Verification items for the finished model (mm, model axes). A direction names the side the tool comes from. Coordinates: 2 decimals unless noted, no trailing zeros. Order: outer loops, then holes, each group sorted by start corner. A loop starts at its lowest first (then second) coordinate and runs counter-clockwise, first axis right, second up. Notation, with made-up numbers: M 34.5,-11.5 L 61.5,-11.5 A8 ccw 61.5,-2.5 Z; hole C -30,74.5 d5. An arc over 180 degrees is marked long. Return JSON: item names as keys, results as strings. Group by question number.
1. Material ranges on line 1 along Y through (x, z) = (0, 12.15); line 2 along X through (y, z) = (4, 2.25); line 3 along X through (y, z) = (0, 11.5), recorded low to high.
2. Section check D-D, the plane z = 10. Record the cut outline in (x, y), plus the area to 3 significant figures.
3. Gauge pin test, flat ends, axial feed: pin 1 (2.5 mm diameter, centred on y = 0, z = 7.5, fed in from -X); pin 2 (2 mm diameter, centred on x = -3.5, z = 11.5, fed in from +Y); pin 3 (1.5 mm diameter, centred on x = -2, y = 8, fed in from +Z). Record the tip position at first contact, or that the pin passes through.
4. Section check A-A, the plane y = 0. Record the cut outline in (x, z), plus the area to 3 significant figures.
5. Section check C-C, the plane z = 7. Record the cut outline in (x, y).
6. Mould release check, pull along X, two halves, no side actions. Record for faces 1 (the conical face through (1.409, 3.399, 12.636)), 2 (the flat face through (1.3, 1.3, 13)), 3 (the flat face through (1.361, -2.314, 7.479)): +X half, -X half, draft (parallel to the pull), parting line (faces both ways), or undercut.
7. Section check B-B, the plane z = 1.75. Record the cut outline in (x, y).
8. Set-up check for faces 4 (the flat face through (1.32, 2.34, 7.48)), 5 (the cylindrical face through (0.97, -1.27, 10.97)): record each of +Z, -Z, +X, -X, +Y, -Y from which the full face is reachable in a straight line by a thin tool's end or side.
```python
from build123d import *

# Parameters (mm, degrees)
SKETCH_W        = 12
SKETCH_H        = 12
POCKET_DEPTH    = 6
POCKET001_DEPTH = 3


with BuildPart() as part:
    # Sketch002 → Revolution (revolve)
    with BuildSketch(Plane.YZ):
        Polygon((1.6, 13), (1.6, 0), (17, 0), (17, 5.5), (3, 13), align=None)
    revolve(axis=Axis((0, 0, 0), (0, 0, 1)))

    # Sketch (on Face2 of Revolution) → Pocket (cut)
    with BuildSketch(Plane.YX):
        Rectangle(SKETCH_W, SKETCH_H)
    extrude(amount=-POCKET_DEPTH, mode=Mode.SUBTRACT)

    # Sketch003 (on Face2 of Pocket) → Pocket001 (cut)
    with BuildSketch(Plane.YX.offset(-6)):
        Polygon((3.1, 0), (1.55, 2.684679), (-1.55, 2.684679), (-3.1, 0), (-1.55, -2.684679), (1.55, -2.684679), align=None)
    extrude(amount=-POCKET001_DEPTH, mode=Mode.SUBTRACT)


solid = part.part
```
Answers follow:
{
 "1": {"line 1": "-4.59 to -1.6, 1.6 to 4.59", "line 2": "-16.52 to -6, 6 to 16.52", "line 3": "-5.8 to -1.6, 1.6 to 5.8"},
 "2": {"outline": "C 0,0 d17.2; hole C 0,0 d3.2", "area": "224 mm^2"},
 "3": {"pin 1": "x = -15.6", "pin 2": "y = 6.88", "pin 3": "z = 10.59"},
 "4": {"outline": "M -17,0 L -6,0 L -6,6 L -2.68,6 L -2.68,9 L -1.6,9 L -1.6,13 L -3,13 L -17,5.5 Z; M 1.6,9 L 2.68,9 L 2.68,6 L 6,6 L 6,0 L 17,0 L 17,5.5 L 3,13 L 1.6,13 Z", "area": "236 mm^2"},
 "5": {"outline": "C 0,0 d28.4; hole M -2.68,-1.55 L 0,-3.1 L 2.68,-1.55 L 2.68,1.55 L 0,3.1 L -2.68,1.55 Z"},
 "6": {"face 1": "parting line", "face 2": "draft", "face 3": "undercut"},
 "7": {"outline": "C 0,0 d34; hole M -6,-6 L 6,-6 L 6,6 L -6,6 Z"},
 "8": {"face 4": "-Z", "face 5": "+Z, -Z"}
}
